Verification items for the finished model (mm, model axes). A direction names the side the tool comes from. Coordinates: 2 decimals unless noted, no trailing zeros. Loops run counter-clockwise (first coordinate to the right, second up) from the corner with the lowest first, then second, coordinate; pieces in that order, holes last. Notation, with made-up numbers: (-10.5, 33) -> (20.5, 33) arc R20 cw to (20.5, 71) -> close; hole circle Ø3 at (29.5, 88). An arc over 180 degrees is marked (long way). Write item = value, one per line.
```python
from build123d import *

# Parameters (mm, degrees)
F1_DEPTH = 127
F2_W     = 89.568419
F2_H     = 63.5
F3_DEPTH = 215.9
F4_R     = 15.875
F5_DEPTH = 139.7


with BuildPart() as f1:
    # F0 (on Top) → F1 (new body)
    with BuildSketch(Plane.XY):
        Polygon((44.45, 25.663219), (-44.45, 25.663219), (0, -51.326439), align=None)
    extrude(amount=F1_DEPTH)

    # F2 (on Top) → F3 (intersect)
    with BuildSketch(Plane.XY):
        with Locations((-0.249351, -5.168639)):
            Rectangle(F2_W, F2_H)
    extrude(amount=F3_DEPTH, mode=Mode.INTERSECT)

    # F4 (on Top) → F5 (join)
    with BuildSketch(Plane.XY):
        Circle(F4_R)
    extrude(amount=F5_DEPTH)


solid = f1.part
```
1) Material ranges on line 1 (Z direction, x = -12, y = -30); line 2 (X direction, y = -34, z = 20); line 3 (X direction, y = -15.5, z = 72), recorded low to high.
Ans:
line_1 = 0 to 127
line_2 = -10 to 10
line_3 = -20.68 to 20.68
2) Depth check by flat-ended pin: pin 1 Ø4 at (y, z) = (-7, 43) entering from -X; pin 2 Ø5 at (y, z) = (17.5, 64) entering from +X; pin 3 Ø1 at (y, z) = (-12, 57.5) entering from -X. Enter the tip coordinate at first touch or a pass-through.
Ans:
pin_1 = -26.75
pin_2 = 41.18
pin_3 = -22.99
3) Tool access check on faces 1 (the face through (26.13, -6.07, 62.61)), 2 (the face through (-3.441, -15.497, 133.261)). Record the directions out of +Z, -Z, +X, -X, +Y, -Y that give a thin tool (end or side, any length) a straight path to the whole face; none if there is none.
Ans:
face_1 = +Z, -Z, +X, -Y
face_2 = +Z
4) Sectioned sample at C-C, the plane z = 121. Record the cut outline in (x, y).
Ans:
outline = (-44.45, 25.66) -> (-8.32, -36.92) -> (8.32, -36.92) -> (44.45, 25.66) -> close
5) Sectioned sample at B-B, the plane y = 9.5. Record the cut outline in (x, z), plus the area to 3 significant figures.
Ans:
outline = (-35.12, 0) -> (35.12, 0) -> (35.12, 127) -> (12.72, 127) -> (12.72, 139.7) -> (-12.72, 139.7) -> (-12.72, 127) -> (-35.12, 127) -> close
area = 9,240 mm2
6) Sectioned sample at A-A, the plane x = 0. Record the cut outline in (y, z) (3 decimals).
Ans:
outline = (-36.919, 0) -> (25.663, 0) -> (25.663, 127) -> (15.875, 127) -> (15.875, 139.7) -> (-15.875, 139.7) -> (-15.875, 127) -> (-36.919, 127) -> close
7) Sectioned sample at D-D, the plane x = -32. Record the cut outline in (y, z).
Ans:
outline = (4.1, 0) -> (25.66, 0) -> (25.66, 127) -> (4.1, 127) -> close
